```python
from build123d import *

# Parameters (mm, degrees)
SKETCH_1_R      = 2.5
EXTRUDE_1_DEPTH = 5


with BuildPart() as part:
    # 草图1 → 凸台-拉伸1 (new body)
    with BuildSketch(Plane(origin=(0, 0, 0), x_dir=(1, 0, 0), z_dir=(0, 1, 0))):
        with BuildLine():
            Line((20, 21), (30, 21))
            Line((30, 21), (30, 13))
            Line((30, 13), (37, 13))
            Line((37, 13), (37, 14))
            Line((37, 14), (38, 14))
            Line((38, 14), (38, 9))
            Line((38, 9), (37, 9))
            Line((37, 9), (37, 10))
            Line((37, 10), (30, 10))
            Line((30, 10), (30, 8))
            ThreePointArc((30, 8), (29.121320344, 5.878679656), (27, 5))
            Line((27, 5), (26.206359593, 5))
            ThreePointArc((26.206359593, 5), (24.165118141, 5.435645354), (22.47957963, 6.666666667))
            ThreePointArc((22.47957963, 6.666666667), (15.026019705, 10), (7.57245978, 6.666666667))
            ThreePointArc((7.57245978, 6.666666667), (5.88692127, 5.435645354), (3.845679818, 5))
            Line((3.845679818, 5), (3, 5))
            ThreePointArc((3, 5), (0.878679656, 5.878679656), (0, 8))
            Line((0, 8), (0, 10))
            Line((0, 10), (-7, 10))
            Line((-7, 10), (-7, 9))
            Line((-7, 9), (-8, 9))
            Line((-8, 9), (-8, 14))
            Line((-8, 14), (-7, 14))
            Line((-7, 14), (-7, 13))
            Line((-7, 13), (0, 13))
            Line((0, 13), (0, 21))
            Line((0, 21), (10, 21))
            Line((10, 21), (10, 16))
            Line((10, 16), (20, 16))
            Line((20, 16), (20, 21))
        make_face()
        with Locations(Location((5, 10, 0), (0, 0, 270))):
            Circle(SKETCH_1_R, mode=Mode.SUBTRACT)
        with Locations(Location((25, 10, 0), (0, 0, 270))):
            Circle(SKETCH_1_R, mode=Mode.SUBTRACT)
    extrude(amount=EXTRUDE_1_DEPTH)


solid = part.part
```
CAD build for the part. Positions are in the model's coordinates, mm. A direction names the side the tool comes from. Give positions to 0.01 mm unless a question says otherwise; leave off trailing zeros. Order: outer loops, then holes, each group sorted by start corner. A loop starts at its lowest first (then second) coordinate and runs counter-clockwise, first axis right, second up.
(1) Drill centre lines: L1, parallel to X at y = 1.05, z = -8.5; L2, parallel to X at y = 1.95, z = -16.5; L3, parallel to Z at x = 34.5, y = 4.55. Where is each one in solid material? Low to high.
(2) Saw through at D-D, the plane x = 32. Give the cut face in (y, z), then the cut area to 3 significant figures.
(3) Flat gauge pins, fed straight in: pin 1 (2.5 mm diameter, centred on x = 35, y = 2.5, fed in from -Z); pin 2 (1.5 mm diameter, centred on y = 1.5, z = -15.5, fed in from +X); pin 3 (1.5 mm diameter, centred on y = 2.5, z = -17, fed in from -X); pin 4 (1 mm diameter, centred on x = 5, z = -8.5, fed in from +Y). Where does each tip first touch, or does it go through?
(4) Tool access for faces 5 (the flat face through (37, 2.5, -13.5)), 6 (the flat face through (37.5, 2.5, -9)), 7 (the flat face through (-7, 2.5, -9.5)), 8 (the flat face through (5, 2, -21)): list every direction of +Z, -Z, +X, -X, +Y, -Y with a clear straight run to the whole face (end or side of a thin tool).
(5) Mould opens along Z. For faces 1 (the flat face through (15, 0, -13)), 2 (the cylindrical face through (27.48, 2.46, -10.33)), 3 (the cylindrical face through (5.1, 2.5, -12.5)), 4 (the flat face through (-7.5, 2.5, -14)) say: released by +Z, released by -Z, zero draft, split by the parting line, or undercut.
(6) Saw through at A-A, the plane y = 1.05. State how many separate pieces and enclosed holes the cut face has, then the cut area to 3 significant figures.
(7) Saw through at B-B, the plane z = -6.25. Give the cut face in (x, y), then the cut area to 3 significant figures.
(8) Saw through at C-C, the plane x = 5. Give the cut face in (y, z).
Results found:
1. L1: x = 0 to 3, 7 to 9.76, 20.29 to 23, 27 to 30
1. L2: x = 0 to 10, 20 to 30
1. L3: z = -13 to -10
2. outline: (0, -13) - (5, -13) - (5, -10) - (0, -10) - close
2. area: 15.0 mm2
3. pin 1: stops at z = -13
3. pin 2: stops at x = 30
3. pin 3: stops at x = 0
3. pin 4: passes through
4. face 5: -Z, +Y, -Y
4. face 6: +Z, +X, +Y, -Y
4. face 7: +Z, +Y, -Y
4. face 8: -Z, +X, -X, +Y, -Y
5. face 1: zero draft
5. face 2: undercut
5. face 3: undercut
5. face 4: released by -Z
6. separate pieces: 1
6. enclosed holes: 2
6. area: 376 mm2
7. outline: (0.56, 0) - (7.15, 0) - (7.15, 5) - (0.56, 5) - close; (22.9, 0) - (29.44, 0) - (29.44, 5) - (22.9, 5) - close
7. area: 65.6 mm2
8. outline: (0, -21) - (5, -21) - (5, -12.5) - (0, -12.5) - close; (0, -7.5) - (5, -7.5) - (5, -5.14) - (0, -5.14) - close
